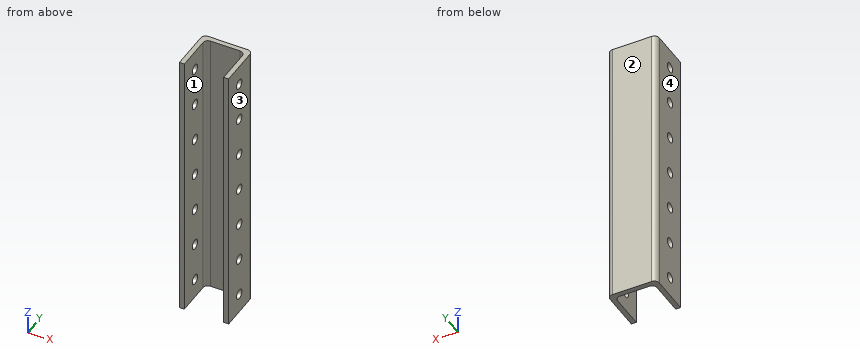
Autodesk Inventor part; units mm, degrees
ref_plane "YZ Plane" through (0, 0, 0) normal (1, 0, 0) x (0, 1, 0)
ref_plane "XZ Plane" through (0, 0, 0) normal (0, 1, 0) x (-1, 0, 0)
ref_plane "XY Plane" through (0, 0, 0) normal (0, 0, 1) x (1, 0, 0)
sketch "Sketch1" plane through (0, 0, 0) normal (0, 0, 1) x (1, 0, 0)
  line L0 (-15.875, 0) -> (-12.7, 0)
  line L1 (-12.7, 0) -> (-12.7, 22.352)
  line L2 (-9.525, 25.527) -> (9.525, 25.527)
  line L3 (12.7, 22.352) -> (12.7, 0)
  line L4 (12.7, 0) -> (15.875, 0)
  line L5 (15.875, 0) -> (15.875, 25.527)
  line L6 (12.7, 28.702) -> (-12.7, 28.702)
  line L7 (-15.875, 25.527) -> (-15.875, 0)
  arc A0 (-9.525, 25.527) -> (-12.7, 22.352) centre (-9.525, 22.352) ccw
  arc A1 (12.7, 22.352) -> (9.525, 25.527) centre (9.525, 22.352) ccw
  arc A2 (-12.7, 28.702) -> (-15.875, 25.527) centre (-12.7, 25.527) ccw
  arc A3 (15.875, 25.527) -> (12.7, 28.702) centre (12.7, 25.527) ccw
  line L8 (0, 35.2315) -> (0, -5.8719)
  point P0 (0, 0)
  dimension "d0" = 28.702
  dimension "d1" = 31.75
  dimension "d2" = 3.175
  dimension "d3" = 3.175
  dimension "d4" = 3.175
extrude "Extrusion1" add sketch "Sketch1" along normal mid plane 177.8
sketch "Sketch4" plane through (15.875, 0, 88.9) normal (1, 0, 0) x (0, 0, -1)
  line L0 (88.9, -5.7404) -> (88.9, 34.4424) construction
  line L1 (-35.56, 0) -> (213.36, 0) construction
  circle A0 centre (88.9, 12.7) radius 3.175
  point P0 (88.9, 0)
  dimension "d34" = 12.7
  dimension "d35" = 0
  dimension "d36" = 6.35
extrude "Extrusion4" cut sketch "Sketch4" against normal up to surface (31.75 mm away)
pattern_linear "Rectangular Pattern3" count 30 spacing 25.4 along (0, 0, 1) count 30 spacing 25.4 along (0, 0, -1) of "Extrusion4"
equation "\"d5\" = ExtensionLen"
equation "\"ExtensionLen\" = 177.8"
properties part number "NTowerChannelBracket" material "Aluminum 6061"
Geometry: final body of the model. Coordinates: model frame, mm. Face numbers are marked on the shaded views. Give positions to 0.01 mm unless a question says otherwise; leave off trailing zeros. Order: outer loops, then holes, each group sorted by start corner. A loop starts at its lowest first (then second) coordinate and runs counter-clockwise, first axis right, second up. Notation, with made-up numbers: (54, -8) -> (87, -8) arc R31 ccw to (87, 31) -> close; hole circle Ø2 at (-24.75, 50). An arc over 180 degrees is marked (long way). Answer as a JSON object with one key per item and string values.
Q1. Section D-D (x = 11). Output: boundary loops of the cut face in (y, z), plus the area to 3 significant figures.
Entries:
{"outline": "(25.16, -88.9) -> (28.7, -88.9) -> (28.7, 88.9) -> (25.16, 88.9) -> close", "area": "629 mm^2"}
Q2. Section C-C (x = 4). Output: boundary loops of the cut face in (y, z), plus the area to 3 significant figures.
Entries:
{"outline": "(25.53, -88.9) -> (28.7, -88.9) -> (28.7, 88.9) -> (25.53, 88.9) -> close", "area": "565 mm^2"}
Q3. Section B-B (y = 12.7). State how many separate pieces and enclosed holes the cut face has, plus the area to 3 significant figures.
Entries:
{"separate pieces": "16", "enclosed holes": "0", "area": "847 mm^2"}
Q4. First-contact query: pin 1 (4 mm diameter, centred on x = 5, y = 25, fed in from -Z); pin 2 (1 mm diameter, centred on x = -5.5, z = 23.5, fed in from -Y). Flat tips, straight axial feed; report the tip coordinate or a pass-through.
Entries:
{"pin 1": "stops at z = -88.9", "pin 2": "stops at y = 25.53"}
Q5. Section A-A (z = 50.8). Output: boundary loops of the cut face in (x, y) (3 decimals), plus the area to 3 significant figures.
Entries:
{"outline": "(-15.875, 0) -> (-12.7, 0) -> (-12.7, 9.525) -> (-15.875, 9.525) -> close; (-15.875, 15.875) -> (-12.7, 15.875) -> (-12.7, 22.352) arc R3.175 cw to (-9.525, 25.527) -> (9.525, 25.527) arc R3.175 cw to (12.7, 22.352) -> (12.7, 15.875) -> (15.875, 15.875) -> (15.875, 25.527) arc R3.175 ccw to (12.7, 28.702) -> (-12.7, 28.702) arc R3.175 ccw to (-15.875, 25.527) -> close; (12.7, 0) -> (15.875, 0) -> (15.875, 9.525) -> (12.7, 9.525) -> close", "area": "223 mm^2"}
Q6. Draft query along X for the marked faces 1, 2, 3 and 4. Return one class per face: released by +X, released by -X, zero draft, split by the parting line, or undercut.
Entries:
{"face 1": "undercut", "face 2": "zero draft", "face 3": "released by +X", "face 4": "released by -X"}
Q7. Material intervals for probe 1 along X at (y, z) = (9.25, 71.5) (3 decimals); probe 2 along Y at (x, z) = (9, 18); probe 3 along Y at (x, z) = (14.25, -50.8) (3 decimals), sorted ascending.
Entries:
{"probe 1": "x = -15.875 to -12.7, 12.7 to 15.875", "probe 2": "y = 25.53 to 28.7", "probe 3": "y = 0 to 9.525, 15.875 to 28.298"}
